For this review, take the finished solid that the model builds, in its own axes (mm). Give positions to 0.01 mm unless a question says otherwise; leave off trailing zeros. Loops run counter-clockwise (first coordinate to the right, second up) from the corner with the lowest first, then second, coordinate; pieces in that order, holes last. Notation, with made-up numbers: (66, 38.5) -> (90, 38.5) arc R19 cw to (90, 69.5) -> close; hole circle Ø7 at (-5.75, -4.5). An arc over 180 degrees is marked (long way). Answer as CSV lines item,"result". Start each with the question number.
Item 1: Add section B-B on z = -92. State the section outline as (x, y) points.
Item 2: Clearance check with flat-ended pins moving along their axes: P1, Ø1.5, axis at x = 57.5, z = -102, coming from the +Y side; P2, Ø1, axis at y = 3, z = -56, coming from the +X side; P3, Ø1, axis at x = 47.5, y = 2.5, coming from the +Z side; P4, Ø1.2, axis at x = 62.5, y = 2, coming from the -Z side. State where each tip first meets the part, or that it passes through.
Item 3: For L1, parallel to Z at x = 49.5, y = 1.7; L2, parallel to X at y = 1.2, z = -99; L3, parallel to Z at x = 84, y = 2.1, list the stretches that pass through material, from the lowest coordinate up. Write a range as from..to.
Item 4: Add section C-C on x = 78.5. State the section outline as (y, z) points.
Item 5: Add section A-A on y = 1.2. State how many separate pieces and enclosed holes the cut face has, plus the area to 3 significant figures.
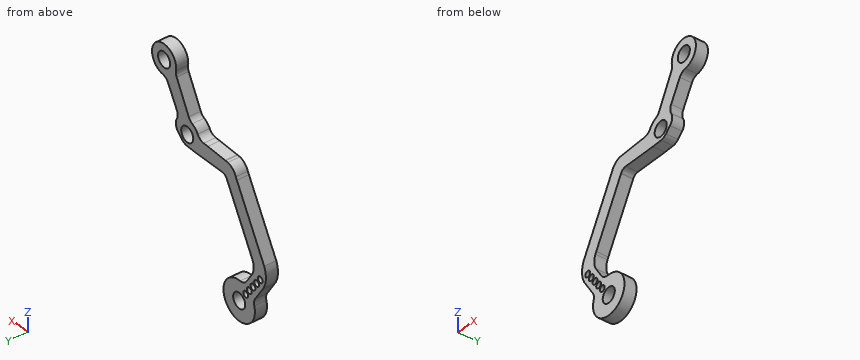
```python
from build123d import *

# Parameters (mm, degrees)
SKETCH2_R           = 2.5
SKETCH2_R_2         = 3.4
BOSS_EXTRUDE1_DEPTH = 4
FILLET1_R           = 3
SKETCH3_R           = 1
CUT_EXTRUDE2_DEPTH  = 4
SKETCH5_W           = 0.9
SKETCH5_H           = 4


with BuildPart() as part:
    # Sketch2 → Boss-Extrude1 (new body)
    with BuildSketch(Plane(origin=(0, 0, 0), x_dir=(1, 0, 0), z_dir=(0, 1, 0))):
        with BuildLine():
            ThreePointArc((49.0624911, 100.728722197), (55.253975507, 111.876765002), (45.278809785, 103.932622106))
            Line((45.278809785, 103.932622106), (41.677103445, 98.359455452))
            Line((41.677103445, 98.359455452), (40.917682236, 97.184351056))
            ThreePointArc((40.917682236, 97.184351056), (40.000914232, 93.684113367), (40.729811239, 90.139986308))
            Line((40.729811239, 90.139986308), (51.995593872, 69.121735128))
            Line((51.995593872, 69.121735128), (52.448751423, 68.276291936))
            ThreePointArc((52.448751423, 68.276291936), (53.733769558, 66.46917356), (55.737555004, 65.519546097))
            Line((55.737555004, 65.519546097), (56.575581952, 65.474059755))
            Line((56.575581952, 65.474059755), (56.904280571, 65.456218685))
            Line((56.904280571, 65.456218685), (64.043852088, 65.068697747))
            Line((64.043852088, 65.068697747), (67.659658755, 64.927019071))
            ThreePointArc((67.659658755, 64.927019071), (68.973857559, 62.514332624), (71.364365032, 61.16020988))
            Line((71.364365032, 61.16020988), (77.3922419, 49.235496946))
            ThreePointArc((77.3922419, 49.235496946), (85.295038859, 43.696471142), (81.278467798, 52.471558808))
            Line((81.278467798, 52.471558808), (75.926202221, 62.342787356))
            ThreePointArc((75.926202221, 62.342787356), (77.117833046, 64.012589982), (77.538655529, 66.020358214))
            Line((77.538655529, 66.020358214), (73.882441794, 69.676571949))
            Line((73.882441794, 69.676571949), (69.341583584, 69.864669723))
            Line((69.341583584, 69.864669723), (65.404712603, 69.864669723))
            Line((65.404712603, 69.864669723), (58.04793187, 69.864669723))
            ThreePointArc((58.04793187, 69.864669723), (56.992330015, 70.157110244), (56.212176606, 70.925990854))
            ThreePointArc((56.212176606, 70.925990854), (56.161986001, 71.014595828), (56.115987655, 71.105447853))
            Line((56.115987655, 71.105447853), (45.913475043, 90.139986308))
            ThreePointArc((45.913475043, 90.139986308), (45.708651409, 90.489699119), (45.530826332, 90.853883157))
            ThreePointArc((45.530826332, 90.853883157), (45.074746145, 93.175228741), (45.661998303, 95.466907026))
            Line((45.661998303, 95.466907026), (49.0624911, 100.728722197))
        make_face()
        with Locations(Location((82.095552315, 47.538773298, 0), (0, 0, 270))):
            Circle(SKETCH2_R, mode=Mode.SUBTRACT)
        with Locations(Location((72.538655529, 66.020358214, 0), (0, 0, 270))):
            Circle(SKETCH2_R, mode=Mode.SUBTRACT)
        with Locations(Location((51.053576092, 106.916256485, 0), (0, 0, 270))):
            Circle(SKETCH2_R_2, mode=Mode.SUBTRACT)
    extrude(amount=BOSS_EXTRUDE1_DEPTH)

    # Fillet1
    fillet1_edges = [part.edges().sort_by_distance(p)[0] for p in [
        (71.364365032, 2, -61.16020988),
        (67.659658755, 2, -64.927019071),
        (45.278809785, 2, -103.932622106),
        (49.0624911, 2, -100.728722197),
        (73.882441794, 2, -69.676571949),
        (77.538655529, 2, -66.020358214),
        (75.926202221, 2, -62.342787356),
        (81.278467798, 2, -52.471558808),
        (77.3922419, 2, -49.235496946),
    ]]
    fillet(fillet1_edges, radius=FILLET1_R)

    # Sketch3 → Cut-Extrude2 (cut)
    with BuildSketch(Plane(origin=(0, 4, 0), x_dir=(1, 0, 0), z_dir=(0, 1, 0))):
        with Locations(Location((48.374282672, 103.36324554, 0), (0, 0, 270))):
            Circle(SKETCH3_R)
        with Locations(Location((46.86906165, 101.367171976, 0), (0, 0, 270))):
            Circle(SKETCH3_R)
        with Locations(Location((45.363840628, 99.371098411, 0), (0, 0, 270))):
            Circle(SKETCH3_R)
        with Locations(Location((43.858619606, 97.375024847, 0), (0, 0, 270))):
            Circle(SKETCH3_R)
        with Locations(Location((42.353398584, 95.378951282, 0), (0, 0, 270))):
            Circle(SKETCH3_R)
    extrude(amount=-CUT_EXTRUDE2_DEPTH, mode=Mode.SUBTRACT)

    # Sweep1: sweep along a path in Sketch4
    with BuildLine(Plane(origin=(0, 4, 0), x_dir=(1, 0, 0), z_dir=(0, 1, 0))) as sweep1_path:
        CenterArc((51.053576092, 106.916256485), 3.4, 0, 360)
    # Sketch5 → Sweep1 (sweep)
    with BuildSketch(Plane(origin=(45.965783702, 0, -109.06060876), x_dir=(0.9214977377283068, 0, 0.38838372695262713), z_dir=(-0.38838372695262713, 0, 0.9214977377283068))):
        with Locations((2.571220706, 2)):
            Rectangle(SKETCH5_W, SKETCH5_H)
    sweep(path=sweep1_path.line)


solid = part.part
```
Computed values:
1,outline,"(40.14, 0) -> (45.17, 0) -> (45.17, 4) -> (40.14, 4) -> close"
2,P1,"through"
2,P2,"x = 79.64"
2,P3,"z = -76.58"
2,P4,"z = -69.86"
3,L1,"-113.23..-108.87, -104.96..-100.26, -83.45..-73.78"
3,L2,"42.09..44.44, 46.29..47.95"
3,L3,"-52.16..-49.16, -45.92..-42.92"
4,outline,"(0, -57.6) -> (4, -57.6) -> (4, -44.06) -> (0, -44.06) -> close"
5,separate pieces,"1"
5,enclosed holes,"8"
5,area,"501 mm²"
